from build123d import *

# Parameters (mm, degrees)
SKETCH_4_W          = 30
SKETCH_4_H          = 20
EXTRUDE_1_DEPTH     = 2
SKETCH_5_W          = 4
SKETCH_5_H          = 20
EXTRUDE_2_DEPTH     = 30
FILLET_1_R          = 10
SKETCH_6_R          = 2.1
CUT_EXTRUDE_2_DEPTH = 30
FILLET_2_R          = 6


with BuildPart() as part:
    # 草图4 → 凸台-拉伸1 (new body)
    with BuildSketch(Plane.XY):
        with Locations((-9.056603774, -12.830188679)):
            Rectangle(SKETCH_4_W, SKETCH_4_H)
    extrude(amount=EXTRUDE_1_DEPTH)

    # 草图5 → 凸台-拉伸2 (add)
    with BuildSketch(Plane.XY.offset(2)):
        with Locations((-9.056603774, -12.830188679)):
            Rectangle(SKETCH_5_W, SKETCH_5_H)
    extrude(amount=EXTRUDE_2_DEPTH)

    # 圆角1
    fillet_1_edges = [part.edges().sort_by_distance(p)[0] for p in [
        (-9.056603774, -2.830188679, 32),
        (-9.056603774, -22.830188679, 32),
    ]]
    fillet(fillet_1_edges, radius=FILLET_1_R - 0.0001)  # a hair under: the kernel refuses the full size

    # 草图6 → 切除-拉伸2 (cut)
    with BuildSketch(Plane.ZY.offset(11.056603774)):
        with Locations(Location((22, -12.830188679, 0), (0, 0, 270))):
            Circle(SKETCH_6_R)
    extrude(amount=-CUT_EXTRUDE_2_DEPTH, mode=Mode.SUBTRACT)

    # 圆角2
    fillet_2_edges = [part.edges().sort_by_distance(p)[0] for p in [
        (-11.056603774, -12.830188679, 2),
        (-7.056603774, -12.830188679, 2),
    ]]
    fillet(fillet_2_edges, radius=FILLET_2_R)


solid = part.part
Model file for the job. Use its own axes, mm. A direction names the side the tool comes from. Give positions to 0.01 mm unless a question says otherwise; leave off trailing zeros. Order: outer loops, then holes, each group sorted by start corner. A loop starts at its lowest first (then second) coordinate and runs counter-clockwise, first axis right, second up. Notation, with made-up numbers: M 10.25,79 L 56.25,79 A19 ccw 56.25,95 Z; hole C 66.25,-34 d4. An arc over 180 degrees is marked long. Put each result on its own line as item: value. Start each with the question number.
(1) Band-saw the part on D-D on x = -17.5. Give the cut face in (y, z).
(2) Tool access for faces 1 (the face through (5.943, -13, 1)), 2 (the face through (-7.057, -13, 17)), 3 (the face through (-11.057, -13, 17)): list every direction of +Z, -Z, +X, -X, +Y, -Y with a clear straight run to the whole face (end or side of a thin tool).
(3) Drill centre lines: L1, parallel to Z at x = 0.25, y = -12.5; L2, parallel to X at y = -16.75, z = 9; L3, parallel to Z at x = -7.75, y = -11.25. Where is each one in solid material? Low to high. Write a range as [from, to].
(4) Band-saw the part on A-A on z = 22.5. Give the cut face in (x, y).
(5) Band-saw the part on C-C on y = -21. Give the cut face in (x, z), then the cut area to 3 significant figures.
(6) Pin check, flat tips, straight feed: pin 1 Ø6 at (y, z) = (-15.5, 20.5) entering from +X; pin 2 Ø1.5 at (x, z) = (-10.5, 23.5) entering from -Y; pin 3 Ø2 at (x, y) = (-19, -13.5) entering from +Z. Stop position of each tip, or through.
(7) Band-saw the part on B-B on y = -12. Give the cut face in (x, z).
Results below:
1. outline: M -22.83,0 L -2.83,0 L -2.83,2 L -22.83,2 Z
2. face 1: +Z, -Z, +X, +Y, -Y
2. face 2: +Z, +X, +Y, -Y
2. face 3: +Z, -X, +Y, -Y
3. L1: z = [0, 2]
3. L2: x = [-11.06, -7.06]
3. L3: z = [0, 20.62], [23.38, 31.87]
4. outline: M -11.06,-22.82 L -7.06,-22.82 L -7.06,-14.87 L -11.06,-14.87 Z; M -11.06,-10.79 L -7.06,-10.79 L -7.06,-2.84 L -11.06,-2.84 Z
5. outline: M -24.06,0 L 5.94,0 L 5.94,2 L -1.06,2 A6 cw -7.06,8 L -7.06,27.77 L -11.06,27.77 L -11.06,8 A6 cw -17.06,2 L -24.06,2 Z
5. area: 179 mm2
6. pin 1: stops at x = -7.06
6. pin 2: stops at y = -22.8
6. pin 3: stops at z = 2
7. outline: M -24.06,0 L 5.94,0 L 5.94,2 L -1.06,2 A6 cw -7.06,8 L -7.06,20.07 L -11.06,20.07 L -11.06,8 A6 cw -17.06,2 L -24.06,2 Z; M -11.06,23.93 L -7.06,23.93 L -7.06,31.97 L -11.06,31.97 Z
